The listing builds one solid part. Answer for the finished solid, in the listing's coordinates (mm). A direction names the side the tool comes from. Coordinates: 2 decimals unless noted, no trailing zeros. Loops run counter-clockwise (first coordinate to the right, second up) from the corner with the lowest first, then second, coordinate; pieces in that order, holes last. Notation, with made-up numbers: M 57,-10 L 61,-10 A26 cw 61,4 Z; hole C 63.5,41 d10. An arc over 180 degrees is marked long. Answer as a JSON object with one key per item and string values. Group by question number.
1. Given pin 1 (1.3 mm diameter, centred on y = 5, z = 22, fed in from -X); pin 2 (0.8 mm diameter, centred on y = 5.5, z = -29.5, fed in from +X); pin 3 (2 mm diameter, centred on x = 25, y = -2.5, fed in from -Z), each flat-ended and moving along its own axis, determine where each tip first touches the part or whether it passes through.
2. A cutting plane is placed at D-D on y = -1.25. Give the vertices of the cut face in (x, z), and give its area (3 significant figures).
3. Determine the mould class of faces 4 (the face through (0, 9.169, 1)), 5 (the face through (-29.566, 5, 25)), 6 (the face through (36.445, -7.721, 0.533)), 7 (the face through (-37.973, 0, 1)) for opening direction X: released by +X, released by -X, zero draft, split by the parting line, or undercut.
4. A cutting plane is placed at C-C on x = -26.5. Give the vertices of the cut face in (y, z), and give its area (3 significant figures).
5. Straight lines are drawn through the part: L1, parallel to X at y = -0.25, z = -18; L2, parallel to X at y = 4, z = 16.5; L3, parallel to Y at x = -7.5, z = -35. For each, find the intervals that lie inside material, in ascending order.
6. A cutting plane is placed at B-B on z = 9.5. Give the vertices of the cut face in (x, y).
7. For faces 1 (the face through (0, 6.35, 25)), 2 (the face through (0, 0, -12.7)), 3 (the face through (36.445, 7.721, -0.533)), determine the directions among +Z, -Z, +X, -X, +Y, -Y from which every point of the face is accessible in a straight line to the end or side of a thin tool.
8. A cutting plane is placed at A-A on z = 24.5. Give the vertices of the cut face in (x, y), and give its area (3 significant figures).
from build123d import *

# Parameters (mm, degrees)
F0_W     = 75.946
F0_H     = 18.3388
F1_DEPTH = 12.7
F2_W     = 75.946
F2_H     = 18.3388
F4_DEPTH = 25.4
F3_W     = 75.946
F3_H     = 18.3388
F5_DEPTH = 25.4
F6_R     = 1.27
F7_R     = 5.08


with BuildPart() as f1:
    # F0 (on Top) → F1 (new body, symmetric)
    with BuildSketch(Plane.XY):
        Rectangle(F0_W, F0_H)
    extrude(amount=F1_DEPTH, both=True)

    # F2 (on face) → F4 (join)
    with BuildSketch(Plane.XY.offset(12.7)):
        Rectangle(F2_W, F2_H)
        with BuildLine():
            Line((-29.5656, 2.956892), (-29.5656, 6.35))
            Line((-29.5656, 6.35), (29.5656, 6.35))
            Line((29.5656, 6.35), (29.5656, 2.956892))
            ThreePointArc((29.5656, 2.956892), (31.8008, 0), (29.5656, -2.956892))
            Line((29.5656, -2.956892), (29.5656, -6.35))
            Line((29.5656, -6.35), (-29.5656, -6.35))
            Line((-29.5656, -6.35), (-29.5656, -2.956892))
            ThreePointArc((-29.5656, -2.956892), (-31.8008, 0), (-29.5656, 2.956892))
        make_face(mode=Mode.SUBTRACT)
    extrude(amount=F4_DEPTH)

    # F3 (on face) → F5 (join)
    with BuildSketch(Plane(origin=(0, 0, -12.7), x_dir=(1, 0, 0), z_dir=(0, 0, -1))):
        Rectangle(F3_W, F3_H)
        with BuildLine():
            Line((-29.5656, 2.956892), (-29.5656, 6.35))
            Line((-29.5656, 6.35), (29.5656, 6.35))
            Line((29.5656, 6.35), (29.5656, 2.956892))
            ThreePointArc((29.5656, 2.956892), (31.8008, 0), (29.5656, -2.956892))
            Line((29.5656, -2.956892), (29.5656, -6.35))
            Line((29.5656, -6.35), (-29.5656, -6.35))
            Line((-29.5656, -6.35), (-29.5656, -2.956892))
            ThreePointArc((-29.5656, -2.956892), (-31.8008, 0), (-29.5656, 2.956892))
        make_face(mode=Mode.SUBTRACT)
    extrude(amount=F5_DEPTH)

    # F6
    f6_edges = [f1.edges().sort_by_distance(p)[0] for p in [
        (-29.5656, 2.956892, 25.4),
        (-29.5656, -2.956892, 25.4),
        (29.5656, -2.956892, 25.4),
        (29.5656, 2.956892, 25.4),
        (-29.5656, -2.956892, -25.4),
        (-29.5656, 2.956892, -25.4),
        (29.5656, 2.956892, -25.4),
        (29.5656, -2.956892, -25.4),
    ]]
    fillet(f6_edges, radius=F6_R)

    # F7
    f7_edges = [f1.edges().sort_by_distance(p)[0] for p in [
        (37.973, -9.1694, 0),
        (37.973, 9.1694, 0),
        (-37.973, -9.1694, 0),
        (-37.973, 9.1694, 0),
    ]]
    fillet(f7_edges, radius=F7_R)


solid = f1.part
From the geometry:
{
 "1": {"pin 1": "stops at x = -37.97", "pin 2": "stops at x = 37.87", "pin 3": "stops at z = -12.7"},
 "2": {"outline": "M -37.97,-38.1 L -31.54,-38.1 L -31.54,-12.7 L 31.54,-12.7 L 31.54,-38.1 L 37.97,-38.1 L 37.97,38.1 L 31.54,38.1 L 31.54,12.7 L -31.54,12.7 L -31.54,38.1 L -37.97,38.1 Z", "area": "2,580 mm²"},
 "3": {"face 4": "zero draft", "face 5": "undercut", "face 6": "released by +X", "face 7": "released by -X"},
 "4": {"outline": "M -9.17,-38.1 L -6.35,-38.1 L -6.35,-12.7 L 6.35,-12.7 L 6.35,-38.1 L 9.17,-38.1 L 9.17,38.1 L 6.35,38.1 L 6.35,12.7 L -6.35,12.7 L -6.35,38.1 L -9.17,38.1 Z", "area": "752 mm²"},
 "5": {"L1": "x = -37.97 to -31.79, 31.79 to 37.97", "L2": "x = -37.97 to -29.57, 29.57 to 37.97", "L3": "y = -9.17 to -6.35, 6.35 to 9.17"},
 "6": {"outline": "M -37.97,-4.09 A5.08 ccw -32.89,-9.17 L 32.89,-9.17 A5.08 ccw 37.97,-4.09 L 37.97,4.09 A5.08 ccw 32.89,9.17 L -32.89,9.17 A5.08 ccw -37.97,4.09 Z"},
 "7": {"face 1": "+Z", "face 2": "-Z", "face 3": "+Z, -Z, +X, +Y"},
 "8": {"outline": "M -37.97,-4.09 A5.08 ccw -32.89,-9.17 L 32.89,-9.17 A5.08 ccw 37.97,-4.09 L 37.97,4.09 A5.08 ccw 32.89,9.17 L -32.89,9.17 A5.08 ccw -37.97,4.09 Z; hole M -30.22,-2.69 A1.27 cw -29.57,-3.8 L -29.57,-6.35 L 29.57,-6.35 L 29.57,-3.8 A1.27 cw 30.22,-2.69 A3.07 ccw 30.22,2.69 A1.27 cw 29.57,3.8 L 29.57,6.35 L -29.57,6.35 L -29.57,3.8 A1.27 cw -30.22,2.69 A3.07 ccw Z", "area": "600 mm²"}
}
